Autodesk Inventor part; units mm, degrees
ref_plane "YZ Plane" through (0, 0, 0) normal (1, 0, 0) x (0, 1, 0)
ref_plane "XZ Plane" through (0, 0, 0) normal (0, 1, 0) x (-1, 0, 0)
ref_plane "XY Plane" through (0, 0, 0) normal (0, 0, 1) x (1, 0, 0)
sketch "Sketch1" plane through (0, 0, 0) normal (0, 1, 0) x (-1, 0, 0)
  line L0 (0, 0) -> (25.4, 0)
  line L1 (25.4, 0) -> (25.4, -50.8)
  line L2 (25.4, -50.8) -> (0, -50.8)
  line L3 (0, -50.8) -> (0, 0)
  line L4 (22.225, -47.625) -> (22.225, -3.175)
  line L5 (22.225, -3.175) -> (3.175, -3.175)
  line L6 (3.175, -3.175) -> (3.175, -47.625)
  line L7 (3.175, -47.625) -> (22.225, -47.625)
  dimension "d0" = 25.4
  dimension "d1" = 50.8
  dimension "d2" = 3.175
extrude "Extrusion1" add sketch "Sketch1" along normal blind 533.4
sketch "Sketch2" plane through (0, 0, 0) normal (1, 0, 0) x (0, 0, -1)
  point P0 (0, 0)
sketch "Sketch3" plane through (0, 0, 0) normal (0, -1, 0) x (1, 0, 0)
  line L0 (-3.175, -47.625) -> (-22.225, -47.625)
  line L1 (-22.225, -47.625) -> (-22.225, -3.175)
  line L2 (-22.225, -3.175) -> (-3.175, -3.175)
  line L3 (-3.175, -3.175) -> (-3.175, -47.625)
  line L4 (0, 0) -> (-25.4, 0)
  line L5 (-25.4, 0) -> (-25.4, -50.8)
  line L6 (-25.4, -50.8) -> (0, -50.8)
  line L7 (0, -50.8) -> (0, 0)
extrude "Extrusion2" add sketch "Sketch3" along normal blind 88.9
sketch "Sketch4" plane through (0, 533.4, 0) normal (0, 1, 0) x (1, 0, 0)
  line L0 (-22.225, 47.625) -> (-3.175, 47.625)
  line L1 (-3.175, 47.625) -> (-3.175, 3.175)
  line L2 (-3.175, 3.175) -> (-22.225, 3.175)
  line L3 (-22.225, 3.175) -> (-22.225, 47.625)
  line L4 (-25.4, 0) -> (0, 0)
  line L5 (0, 0) -> (0, 50.8)
  line L6 (0, 50.8) -> (-25.4, 50.8)
  line L7 (-25.4, 50.8) -> (-25.4, 0)
extrude "Extrusion3" add sketch "Sketch4" along normal blind 88.9
sketch "Sketch6" plane through (0, -88.9, 0) normal (1, 0, 0) x (0, 0, -1)
  line L0 (29.7808, 711.2) -> (29.7808, 547.6875)
  line L1 (50.8, 711.2) -> (50.8, 0)
  line L2 (0, 711.2) -> (50.8, 711.2)
  line L3 (0, 0) -> (0, 711.2)
  line L4 (50.8, 0) -> (0, 0)
  line L5 (0, 0) -> (0, 711.2)
  line L6 (0, 711.2) -> (50.8, 711.2)
  line L7 (50.8, 711.2) -> (50.8, 685.8)
  line L8 (50.8, 685.8) -> (0, 685.8)
  line L9 (0, 685.8) -> (0, 711.2)
  point P0 (0, 88.9)
  dimension "d14" = 25.4
extrude "Extrusion5" cut sketch "Sketch6" against normal blind 25.4 contours L2 L1 L8 L0 | L0 L8 L3 L2
sketch "Sketch7" plane through (0, 596.9, 0) normal (0, 1, 0) x (1, 0, 0)
  line L0 (-3.175, 47.625) -> (-22.225, 47.625)
  line L1 (-3.175, 3.175) -> (-3.175, 47.625)
  line L2 (-22.225, 3.175) -> (-3.175, 3.175)
  line L3 (-22.225, 47.625) -> (-22.225, 3.175)
  line L4 (0, 50.8) -> (0, 0)
  line L5 (-25.4, 50.8) -> (0, 50.8)
  line L6 (-25.4, 0) -> (-25.4, 50.8)
  line L7 (0, 0) -> (-25.4, 0)
  point P0 (0, 0)
extrude "Extrusion6" add sketch "Sketch7" along normal blind 25.4
properties part number "2x1 20in Alluminum.ver1-1111-2019"
The listing builds one solid part. Answer for the finished solid, in the listing's coordinates (mm). A direction names the side the tool comes from. Coordinates: 2 decimals unless noted, no trailing zeros. Write each loop counter-clockwise with the first axis right and the second up, starting at its lowest first coordinate (ties: lowest second). Pieces come first, ordered by that corner, then holes. Notation, with made-up numbers: M 14,7.25 L 21,7.25 A13 cw 21,14.25 Z; hole C -29.75,-31 d8. An arc over 180 degrees is marked long. Write each question's results on one line, items separated by ' | '.
Item 1: The part is cut by section B-B on x = -9.5. Determine the outline of the cut face in (y, z) (3 decimals).
Answer below:
outline: M -88.9,-50.8 L 622.3,-50.8 L 622.3,-47.625 L -88.9,-47.625 Z; M -88.9,-3.175 L 622.3,-3.175 L 622.3,0 L -88.9,0 Z
Item 2: For a pull along X with two mould halves and no side action, classify faces 3 (the face through (-25.4, 262, -25)), 4 (the face through (-23, 622.3, -24)), 5 (the face through (0, 262, -26)), 6 (the face through (-22.225, 262, -26)) as released by +X, released by -X, zero draft, split by the parting line, or undercut.
Answer below:
face 3: released by -X | face 4: zero draft | face 5: released by +X | face 6: undercut
Item 3: Consider probe 1 along X at (y, z) = (567, -42) (3 decimals); probe 2 along Z at (x, y) = (-12, 71.5) (3 decimals). Determine where each line is inside the solid, lowest interval first. Write a range as [from, to].
Answer below:
probe 1: [-25.4, -22.225], [-3.175, 0] | probe 2: [-50.8, -47.625], [-3.175, 0]
Item 4: The part is cut by section A-A on z = -19. Determine the outline of the cut face in (x, y) (3 decimals), and give its area (3 significant figures).
Answer below:
outline: M -25.4,-88.9 L -22.225,-88.9 L -22.225,622.3 L -25.4,622.3 Z; M -3.175,-88.9 L 0,-88.9 L 0,622.3 L -3.175,622.3 Z | area: 4,520 mm2
Item 5: The part is cut by section C-C on y = 470. Determine the outline of the cut face in (x, z) (3 decimals), and give its area (3 significant figures).
Answer below:
outline: M -25.4,-50.8 L 0,-50.8 L 0,0 L -25.4,0 Z; hole M -22.225,-47.625 L -3.175,-47.625 L -3.175,-3.175 L -22.225,-3.175 Z | area: 444 mm2
Item 6: Which of the six approach directions +Z, -Z, +X, -X, +Y, -Y give full straight-line access (tool end or side, diameter ignored) to faces 1 (the face through (-23, -88.9, -27)), 2 (the face through (-13, 262, -47.625))?
Answer below:
face 1: +Z, -Z, +X, -X, -Y | face 2: +Y, -Y
